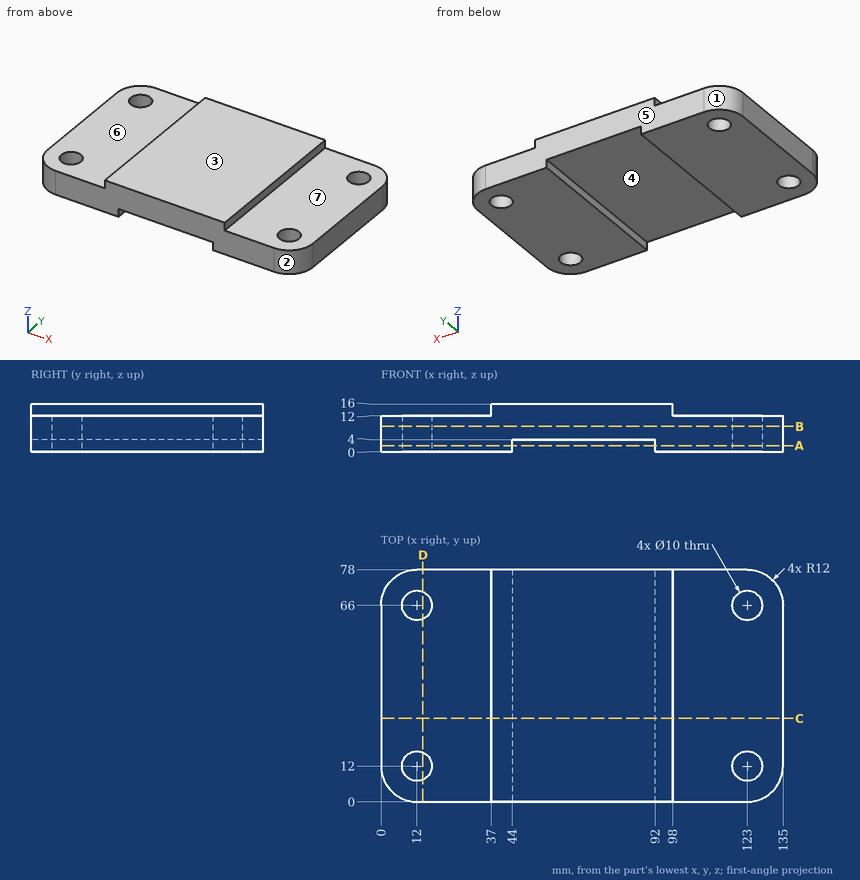
Check sheet for the drawn part. Datum: minimum x, y, z corner. Units: mm. A direction names the side the tool comes from. Coordinates: 2 decimals unless noted, no trailing zeros. Order: outer loops, then holes, each group sorted by start corner. A loop starts at its lowest first (then second) coordinate and runs counter-clockwise, first axis right, second up. Notation, with made-up numbers: (63, 86.5) -> (115, 86.5) arc R21 ccw to (115, 102.5) -> close; hole circle Ø8 at (-2, 72). An arc over 180 degrees is marked (long way). Use a Markdown table: item, result. Add a question column.
1. Cross-section at D-D (x = 14). Enter the section's corners in (y, z), and give its area (3 significant figures).
2. Go/stop test with flat-tipped pins: pin 1 Ø14.5 at (x, y) = (57, 27.5) entering from -Z; pin 2 Ø10 at (x, y) = (21.5, 31.5) entering from +Z; pin 3 Ø4.5 at (y, z) = (36.5, 14.5) entering from +X; pin 4 Ø6 at (x, y) = (123, 66) entering from +Z. Record where each tip stops, or that it passes through.
3. Cross-section at C-C (y = 28). Enter the section's corners in (x, z), and give its area (3 significant figures).
4. Set-up check for the marked faces 5, 6 and 7: record each of +Z, -Z, +X, -X, +Y, -Y from which the full face is reachable in a straight line by a thin tool's end or side.
5. Material ranges on L1, parallel to Y at x = 12, z = 6.5; L2, parallel to X at y = 12, z = 4.25; L3, parallel to X at y = 66, z = 3.75, recorded low to high.
6. Cross-section at A-A (z = 2). Enter the section's corners in (x, y).
7. Cross-section at B-B (z = 8.5). Enter the section's corners in (x, y), and give its area (3 significant figures).
8. Mould release check, pull along X, two halves, no side actions. Record for the marked faces 1, 2, 3 and 4: pulls with the +X half, pulls with the -X half, needs draft (parallel to the pull), parting line crosses it, or undercut.
Filled sheet:
| question | item | result |
|---|---|---|
| 1 | outline | (0, 0) -> (7.42, 0) -> (7.42, 12) -> (0, 12) -> close; (16.58, 0) -> (61.42, 0) -> (61.42, 12) -> (16.58, 12) -> close; (70.58, 0) -> (78, 0) -> (78, 12) -> (70.58, 12) -> close |
| 1 | area | 716 mm2 |
| 2 | pin 1 | z = 4 |
| 2 | pin 2 | z = 12 |
| 2 | pin 3 | x = 98 |
| 2 | pin 4 | through |
| 3 | outline | (0, 0) -> (44, 0) -> (44, 4) -> (92, 4) -> (92, 0) -> (135, 0) -> (135, 12) -> (98, 12) -> (98, 16) -> (37, 16) -> (37, 12) -> (0, 12) -> close |
| 3 | area | 1,670 mm2 |
| 4 | face 5 | +Z, -Z, +X, -X, +Y |
| 4 | face 6 | +Z, -X, +Y, -Y |
| 4 | face 7 | +Z, +X, +Y, -Y |
| 5 | L1 | 0 to 7, 17 to 61, 71 to 78 |
| 5 | L2 | 0 to 7, 17 to 118, 128 to 135 |
| 5 | L3 | 0 to 7, 17 to 44, 92 to 118, 128 to 135 |
| 6 | outline | (0, 12) arc R12 ccw to (12, 0) -> (44, 0) -> (44, 78) -> (12, 78) arc R12 ccw to (0, 66) -> close; (92, 0) -> (123, 0) arc R12 ccw to (135, 12) -> (135, 66) arc R12 ccw to (123, 78) -> (92, 78) -> close; hole circle Ø10 at (12, 12); hole circle Ø10 at (12, 66); hole circle Ø10 at (123, 12); hole circle Ø10 at (123, 66) |
| 7 | outline | (0, 12) arc R12 ccw to (12, 0) -> (123, 0) arc R12 ccw to (135, 12) -> (135, 66) arc R12 ccw to (123, 78) -> (12, 78) arc R12 ccw to (0, 66) -> close; hole circle Ø10 at (12, 12); hole circle Ø10 at (12, 66); hole circle Ø10 at (123, 12); hole circle Ø10 at (123, 66) |
| 7 | area | 10,100 mm2 |
| 8 | face 1 | pulls with the -X half |
| 8 | face 2 | pulls with the +X half |
| 8 | face 3 | needs draft |
| 8 | face 4 | undercut |
